Input: part model. Units: mm. Frame: model coordinates. A direction names the side the tool comes from. Coordinates: 2 decimals unless noted, no trailing zeros. Order: outer loops, then holes, each group sorted by start corner. A loop starts at its lowest first (then second) coordinate and runs counter-clockwise, first axis right, second up. Notation, with made-up numbers: (58, 47.25) -> (68, 47.25) arc R11 ccw to (68, 59.25) -> close; hole circle Ø2 at (-33, 15.5). An arc over 180 degrees is marked (long way). Answer as CSV lines item,"result".
from build123d import *

# Parameters (mm, degrees)
SKETCH_W        = 30
SKETCH_H        = 31.5
PAD_DEPTH       = 1.5
SKETCH001_R     = 2.5
POCKET_DEPTH    = 1.501
SKETCH002_W     = 30
SKETCH002_H     = 1.5
PAD001_DEPTH    = 30
SKETCH003_R     = 2.5
POCKET001_DEPTH = 1.501


with BuildPart() as part:
    # Sketch → Pad (new body)
    with BuildSketch(Plane.XZ):
        with Locations((15, 15.75)):
            Rectangle(SKETCH_W, SKETCH_H)
    extrude(amount=PAD_DEPTH)

    # Sketch001 (on Face6 of Pad) → Pocket (cut, through all)
    with BuildSketch(Plane.XZ.offset(1.5)):
        with Locations((22, 10)):
            Circle(SKETCH001_R)
        with Locations((9, 23)):
            Circle(SKETCH001_R)
    extrude(amount=-POCKET_DEPTH, mode=Mode.SUBTRACT)

    # Sketch002 (on Face4 of Pocket) → Pad001 (join)
    with BuildSketch(Plane(origin=(0, 0, 0), x_dir=(1, 0, 0), z_dir=(0, 1, 0))):
        with Locations((15, -0.75)):
            Rectangle(SKETCH002_W, SKETCH002_H)
    extrude(amount=PAD001_DEPTH)

    # Sketch003 (on Face13 of Pad001) → Pocket001 (cut, through all)
    with BuildSketch(Plane(origin=(0, 0, 1.5), x_dir=(-1, 0, 0), z_dir=(0, 0, 1))):
        with Locations((-9, -9)):
            Circle(SKETCH003_R)
        with Locations((-22, -22)):
            Circle(SKETCH003_R)
    extrude(amount=-POCKET001_DEPTH, mode=Mode.SUBTRACT)


solid = part.part
1. Cut plane D-D (x = 18.5). Return the cut outline in (y, z).
Findings:
outline,"(-1.5, 0) -> (30, 0) -> (30, 1.5) -> (0, 1.5) -> (0, 31.5) -> (-1.5, 31.5) -> close"
2. Mould query, pull axis X, two halves, no side actions, for faces 3 (the face through (8.67, -0.76, 25.48)), 4 (the face through (15, 15, 1.5)), 5 (the face through (30, -1, 9)), 6 (the face through (9.54, 11.44, 0.76)). Classes: released by +X, released by -X, zero draft, split by the parting line, or undercut.
Findings:
face 3,"undercut"
face 4,"zero draft"
face 5,"released by +X"
face 6,"undercut"
3. Cut plane A-A (z = 11.5). Return the cut outline in (x, y).
Findings:
outline,"(0, -1.5) -> (20, -1.5) -> (20, 0) -> (0, 0) -> close; (24, -1.5) -> (30, -1.5) -> (30, 0) -> (24, 0) -> close"
4. Cut plane C-C (y = 22). Return the cut outline in (x, z).
Findings:
outline,"(0, 0) -> (19.5, 0) -> (19.5, 1.5) -> (0, 1.5) -> close; (24.5, 0) -> (30, 0) -> (30, 1.5) -> (24.5, 1.5) -> close"
5. Contact query for flat-ended pins moving along their axis: pin 1 (1.5 mm diameter, centred on x = 7.5, y = 11.5, fed in from +Z); pin 2 (6.5 mm diameter, centred on x = 22, z = 10, fed in from +Y). Output: stop coordinate, or through.
Findings:
pin 1,"stops at z = 1.5"
pin 2,"stops at y = 0"
6. Cut plane B-B (x = 9). Return the cut outline in (y, z), plus the area to 4 significant figures.
Findings:
outline,"(-1.5, 0) -> (6.5, 0) -> (6.5, 1.5) -> (0, 1.5) -> (0, 20.5) -> (-1.5, 20.5) -> close; (-1.5, 25.5) -> (0, 25.5) -> (0, 31.5) -> (-1.5, 31.5) -> close; (11.5, 0) -> (30, 0) -> (30, 1.5) -> (11.5, 1.5) -> close"
area,"77.25 mm2"
7. Ray query, line 1 along Z through (x, y) = (9, -0.45); line 2 along Y through (x, z) = (2, 8.5); line 3 along X through (y, z) = (22, 0.3). Return the intervals inside material, ascending.
Findings:
line 1,"z = 0 to 20.5, 25.5 to 31.5"
line 2,"y = -1.5 to 0"
line 3,"x = 0 to 19.5, 24.5 to 30"
8. Reachability of faces 1 (the face through (15, 0, 17)), 2 (the face through (15, 30, 1)) from +Z, -Z, +X, -X, +Y, -Y: full face, straight path, thin tool, end or side. Return the list, or none.
Findings:
face 1,"+Z, +X, -X, +Y"
face 2,"+Z, -Z, +X, -X, +Y"
